from build123d import *

# Parameters (mm, degrees)
POCKET_DEPTH    = 5
CHAMFER_SIZE    = 0.5
CHAMFER001_SIZE = 0.2


with BuildPart() as part:
    # Sketch → Revolution (revolve)
    with BuildSketch(Plane.XY):
        Polygon((0.5, -10), (1.5, -9), (1.5, 0), (0, 0), (0, -10), align=None)
    revolve(axis=Axis((0, 0, 0), (0, 1, 0)))

    # Sketch001 → Pocket (cut)
    with BuildSketch(Plane.XZ):
        Polygon((0.75, -0.433013), (0.75, 0.433013), (0, 0.866025), (-0.75, 0.433013), (-0.75, -0.433013), (0, -0.866025), align=None)
    extrude(amount=POCKET_DEPTH, mode=Mode.SUBTRACT)

    # Chamfer
    chamfer_edges = [part.edges().sort_by_distance(p)[0] for p in [
        (0.75, -5, 0),
        (0.375, -5, 0.649519),
        (-0.375, -5, 0.649519),
        (-0.75, -5, 0),
        (-0.375, -5, -0.649519),
        (0.375, -5, -0.649519),
    ]]
    chamfer(chamfer_edges, length=CHAMFER_SIZE)

    # Chamfer001
    chamfer001_edges = [part.edges().sort_by_distance(p)[0] for p in [
        (-1.5, 0, 0),
    ]]
    chamfer(chamfer001_edges, length=CHAMFER001_SIZE)


solid = part.part
The model under review builds one solid part; all positions refer to its coordinate system, in mm. A direction names the side the tool comes from. Round coordinates to 2 decimals unless told otherwise and drop trailing zeros. Order: outer loops, then holes, each group sorted by start corner. A loop starts at its lowest first (then second) coordinate and runs counter-clockwise, first axis right, second up. Notation, with made-up numbers: (-37, 88) - (9, 88) arc R17 cw to (9, 100) - close; hole circle Ø2 at (58, 62.5). An arc over 180 degrees is marked (long way). Use one line per item in the form item = value.
Q1. Mouldability with a two-part tool opening along Z and no side actions: class faces 1 (the flat face through (1, 0, 0)), 2 (the cylindrical face through (-1.5, -4.54, -0.07)), 3 (the flat face through (0.75, -2, 0)) as pulls with the +Z half, pulls with the -Z half, needs draft (parallel to the pull), parting line crosses it, or undercut.
Response values:
face_1 = needs draft
face_2 = parting line crosses it
face_3 = undercut
Q2. To check wall thickness, follow line 1 (X direction, y = -0.5, z = -0.05); line 2 (Z direction, x = 0.65, y = -0.75). State the ranges of each line that lie inside material, in increasing order.
Response values:
line_1 = -1.5 to -0.75, 0.75 to 1.5
line_2 = -1.35 to -0.49, 0.49 to 1.35
Q3. Tool access review of faces 4 (the flat face through (-0.75, -2, 0)), 5 (the flat face through (0, -10, 0)): name each direction out of +Z, -Z, +X, -X, +Y, -Y from which nothing blocks a thin tool from reaching the whole face with its end or side.
Response values:
face_4 = +Y
face_5 = +Z, -Z, +X, -X, -Y
Q4. Add section B-B on z = 0. Give the boundary of the cut face in (x, y).
Response values:
outline = (-1.5, -9) - (-0.5, -10) - (0.5, -10) - (1.5, -9) - (1.5, -0.2) - (1.3, 0) - (0.75, 0) - (0.75, -4.5) - (0.25, -5) - (-0.25, -5) - (-0.75, -4.5) - (-0.75, 0) - (-1.3, 0) - (-1.5, -0.2) - close
Q5. Clearance check with a flat-ended pin moving along its axis: P1, Ø1, axis at x = 0.5, z = 1, coming from the -Y side. State where the tip first meets the part, or that it passes through.
Response values:
P1 = -9.88
Q6. Add section A-A on y = -3.5. Give the boundary of the cut face in (x, z).
Response values:
outline = circle Ø3 at (0, 0); hole (-0.75, -0.43) - (0, -0.87) - (0.75, -0.43) - (0.75, 0.43) - (0, 0.87) - (-0.75, 0.43) - close
